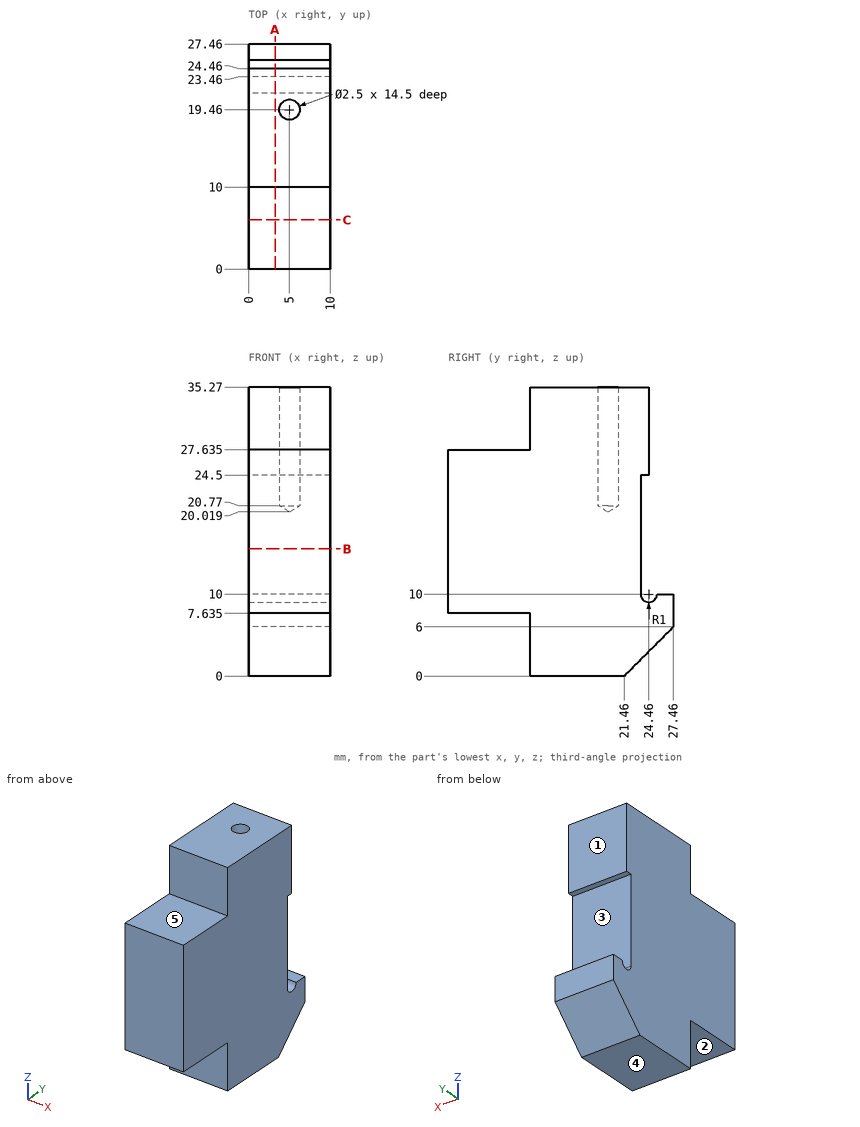
The figure shows three views and two pictorial views of one solid part (mm, origin at its lowest corner). Answer the questions. A direction names the side the tool comes from. Coordinates: 2 decimals unless noted, no trailing zeros. Write each loop counter-clockwise with the first axis right and the second up, starting at its lowest first coordinate (ties: lowest second). Pieces come first, ordered by that corner, then holes. Notation, with made-up numbers: (42.5, 33.25) -> (58.5, 33.25) arc R17 ccw to (58.5, 45.25) -> close; hole circle Ø1 at (-23.75, 30.25). An arc over 180 degrees is marked (long way). Return JSON: item names as keys, results as strings.
(1) The part is cut by section B-B on z = 15.5. Give the vertices of the cut face in (x, y).
Answers below:
{"outline": "(0, 0) -> (10, 0) -> (10, 23.46) -> (0, 23.46) -> close"}
(2) Each of these flat-tipped pins is pushed along its axis until it touches: P1, Ø6, axis at x = 4, z = 33, coming from the -Y side; P2, Ø5, axis at x = 5.5, y = 6.5, coming from the +Z side (3 decimals); P3, Ø3, axis at y = 6.5, z = 20.5, coming from the -X side; P4, Ø1.6, axis at x = 3, y = 26, coming from the +Z side. Where does it stop, or does it pass through?
Answers below:
{"P1": "y = 10", "P2": "z = 27.635", "P3": "x = 0", "P4": "z = 10"}
(3) Consider line 1 along X through (y, z) = (19.46, 25.5); line 2 along Y through (x, z) = (5, 26); line 3 along Y through (x, z) = (5, 24). Determine where each line is inside the solid, lowest interval first. Write a range as from..to.
Answers below:
{"line 1": "0..3.75, 6.25..10", "line 2": "0..18.21, 20.71..24.46", "line 3": "0..18.21, 20.71..23.46"}
(4) The part is cut by section A-A on x = 3.25. Give the vertices of the cut face in (y, z) (3 decimals).
Answers below:
{"outline": "(0, 7.635) -> (10, 7.635) -> (10, 0) -> (21.46, 0) -> (27.46, 6) -> (27.46, 10) -> (25.46, 10) arc R1 cw to (23.46, 10) -> (23.46, 24.5) -> (24.46, 24.5) -> (24.46, 35.27) -> (10, 35.27) -> (10, 27.635) -> (0, 27.635) -> close"}
(5) The part is cut by section C-C on y = 6. Give the vertices of the cut face in (x, z) (3 decimals).
Answers below:
{"outline": "(0, 7.635) -> (10, 7.635) -> (10, 27.635) -> (0, 27.635) -> close"}
(6) Which of the six approach directions +Z, -Z, +X, -X, +Y, -Y give full straight-line access (tool end or side, diameter ignored) to the marked faces 1, 2, 3, 4 and 5?
Answers below:
{"face 1": "+Z, +X, -X, +Y", "face 2": "-Z, +X, -X, -Y", "face 3": "+X, -X, +Y", "face 4": "-Z, +X, -X, +Y, -Y", "face 5": "+Z, +X, -X, -Y"}
